from build123d import *

# Parameters (mm, degrees)
SKETCH1_W                                           = 31.75
SKETCH1_H                                           = 203.2
BOSS_EXTRUDE1_DEPTH                                 = 6.35
SKETCH2_W                                           = 6.35
SKETCH2_H                                           = 41.148
SKETCH2_H_2                                         = 41.91
SKETCH2_W_2                                         = 12.7
SKETCH2_H_3                                         = 4.572
CUT_EXTRUDE1_DEPTH                                  = 7.35
CBORE_FOR_8_BINDING_HEAD_MACHINE_SCREW1_D           = 4.4958
CBORE_FOR_8_BINDING_HEAD_MACHINE_SCREW1_CBORE_D     = 9.525
CBORE_FOR_8_BINDING_HEAD_MACHINE_SCREW1_CBORE_DEPTH = 3.175


with BuildPart() as part:
    # Sketch1 → Boss-Extrude1 (new body)
    with BuildSketch(Plane(origin=(0, 0, 0), x_dir=(1, 0, 0), z_dir=(0, 1, 0))):
        with Locations((15.875, 101.6)):
            Rectangle(SKETCH1_W, SKETCH1_H)
    extrude(amount=BOSS_EXTRUDE1_DEPTH)

    # Sketch2 → Cut-Extrude1 (cut, through all)
    with BuildSketch(Plane(origin=(0, 6.35, 0), x_dir=(1, 0, 0), z_dir=(0, 1, 0))):
        with Locations((28.575, 182.626)):
            Rectangle(SKETCH2_W, SKETCH2_H)
        with Locations((28.575, 134.747)):
            Rectangle(SKETCH2_W, SKETCH2_H_2)
        Polygon((31.75, 59.182), (25.4, 59.182), (25.4, 17.272), (19.05, 17.272), (19.05, 8.382), (31.75, 8.382), align=None)
        with Locations((28.575, 86.487)):
            Rectangle(SKETCH2_W, SKETCH2_H_2)
        with Locations((25.4, 2.286)):
            Rectangle(SKETCH2_W_2, SKETCH2_H_3)
    extrude(amount=-CUT_EXTRUDE1_DEPTH, mode=Mode.SUBTRACT)

    # CBORE for #8 Binding Head Machine Screw1 (through all)
    with Locations(Plane(origin=(0, 0, 0), x_dir=(-1, 0, 0), z_dir=(0, -1, 0))):
        with Locations((-12.7, 31.75), (-12.7, 69.85), (-12.7, 184.15)):
            CounterBoreHole(CBORE_FOR_8_BINDING_HEAD_MACHINE_SCREW1_D / 2, CBORE_FOR_8_BINDING_HEAD_MACHINE_SCREW1_CBORE_D / 2, CBORE_FOR_8_BINDING_HEAD_MACHINE_SCREW1_CBORE_DEPTH)


solid = part.part
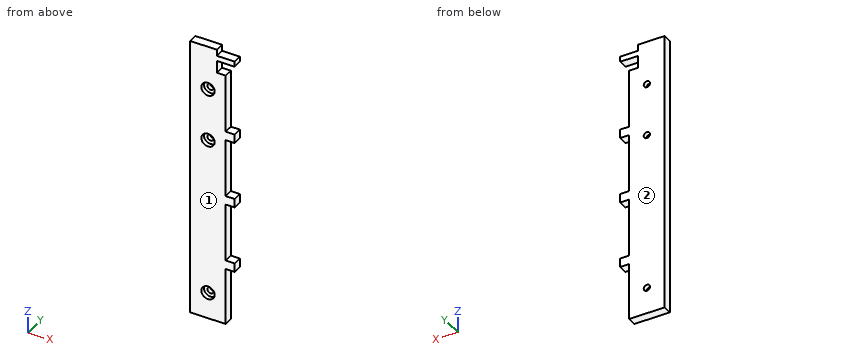
Could you check a few things on this model? Use its own coordinates, in mm. Face numbers are marked on the shaded views. Give positions to 0.01 mm unless a question says otherwise; leave off trailing zeros. Order: outer loops, then holes, each group sorted by start corner. A loop starts at its lowest first (then second) coordinate and runs counter-clockwise, first axis right, second up. Notation, with made-up numbers: (17.25, -12.5) -> (45.25, -12.5) arc R24 cw to (45.25, -1.5) -> close; hole circle Ø9 at (-6, 84). An arc over 180 degrees is marked (long way). Answer in a Markdown table with one row per item. Add a question column.
Item 1: We'd pull the mould along Y, two halves only. Please class the marked faces 1 and 2: pulls with the +Y half, pulls with the -Y half, needs draft (parallel to the pull), parting line crosses it, or undercut.
Item 2: Imagine slicing it at A-A (x = 21). List the corners of the cut face in (y, z) for me.
Item 3: Imagine slicing it at D-D (x = 12.7). Count the separate pieces of the cut face and the enclosed holes in it, and give its area (3 significant figures).
Item 4: I'm going to push flat-ended pins straight in: P1, Ø1.9, axis at y = 4.5, z = -12.5, coming from the +X side; P2, Ø1.9, axis at x = 29.5, y = 4, coming from the -Z side; P3, Ø3.5, axis at y = 2, z = -1.5, coming from the +X side. Where does each tip first touch, or does it pass through?
Item 5: Imagine slicing it at B-B (y = 5). List the corners of the cut face in (x, z) for me.
Item 6: Please list where these lines run through material, in increasing order: probe 1 along Z at (x, y) = (12.7, 1.05); probe 2 along Z at (x, y) = (28, 2.75); probe 3 along X at (y, z) = (1.3, -31.75).
Result:
| question | item | result |
|---|---|---|
| 1 | face 1 | pulls with the -Y half |
| 1 | face 2 | pulls with the +Y half |
| 2 | outline | (0, -203.2) -> (6.35, -203.2) -> (6.35, -17.27) -> (0, -17.27) -> close; (0, -8.38) -> (6.35, -8.38) -> (6.35, -4.57) -> (0, -4.57) -> close |
| 3 | separate pieces | 4 |
| 3 | enclosed holes | 0 |
| 3 | area | 1,160 mm2 |
| 4 | P1 | x = 19.05 |
| 4 | P2 | z = -162.05 |
| 4 | P3 | x = 19.05 |
| 5 | outline | (0, -203.2) -> (25.4, -203.2) -> (25.4, -162.05) -> (31.75, -162.05) -> (31.75, -155.7) -> (25.4, -155.7) -> (25.4, -113.79) -> (31.75, -113.79) -> (31.75, -107.44) -> (25.4, -107.44) -> (25.4, -65.53) -> (31.75, -65.53) -> (31.75, -59.18) -> (25.4, -59.18) -> (25.4, -17.27) -> (19.05, -17.27) -> (19.05, -8.38) -> (31.75, -8.38) -> (31.75, -4.57) -> (19.05, -4.57) -> (19.05, 0) -> (0, 0) -> close; hole circle Ø4.5 at (12.7, -184.15); hole circle Ø4.5 at (12.7, -69.85); hole circle Ø4.5 at (12.7, -31.75) |
| 6 | probe 1 | -203.2 to -188.91, -179.39 to -74.61, -65.09 to -36.51, -26.99 to 0 |
| 6 | probe 2 | -162.05 to -155.7, -113.79 to -107.44, -65.53 to -59.18, -8.38 to -4.57 |
| 6 | probe 3 | 0 to 7.94, 17.46 to 25.4 |
